Could you check a few things on this model? Use its own coordinates, in mm. A direction names the side the tool comes from. Give positions to 0.01 mm unless a question says otherwise; leave off trailing zeros. Order: outer loops, then holes, each group sorted by start corner. A loop starts at its lowest first (then second) coordinate and runs counter-clockwise, first axis right, second up. Notation, with made-up numbers: M -7.5,76 L 4.5,76 A17 cw 4.5,92 Z; hole C 21,-10.5 d6. An arc over 180 degrees is marked long. Use a Markdown table: item, result. Add a question column.
```python
from build123d import *

# Parameters (mm, degrees)
F2_W      = 19
F2_H      = 44
F3_DEPTH  = 23
F3_FACE_W = 19
F3_FACE_H = 44
F4_DEPTH  = 5
F5_R      = 17
F6_T      = -1
F7_R      = 9
F8_DEPTH  = 1
F9_R      = 9
F10_DEPTH = 0.5
F11_R     = 9
F12_DEPTH = 0.5
F14_DEPTH = 25


with BuildPart() as f3:
    # F2 (on offset) → F3 (new body)
    with BuildSketch(Plane.XZ.offset(-25)):
        Rectangle(F2_W, F2_H)
    extrude(amount=F3_DEPTH)

    # F3_face (on face) → F4 (join)
    with BuildSketch(Plane(origin=(0, 25, 0), x_dir=(1, 0, 0), z_dir=(0, 1, 0))):
        Rectangle(F3_FACE_W, F3_FACE_H)
    extrude(amount=F4_DEPTH)

    # F5
    f5_edges = [f3.edges().sort_by_distance(p)[0] for p in [
        (0, 2, 22),
        (0, 2, -22),
    ]]
    fillet(f5_edges, radius=F5_R)

    # F6
    f6_openings = [f3.faces().sort_by_distance(p)[0] for p in [
        (0, 30, 0),
    ]]
    offset(amount=F6_T, openings=f6_openings)

    # F7 (on face) → F8 (cut, symmetric)
    with BuildSketch(Plane(origin=(0, 3, 0), x_dir=(-1, 0, 0), z_dir=(0, 1, 0))):
        Circle(F7_R)
    extrude(amount=F8_DEPTH, both=True, mode=Mode.SUBTRACT)

    # F9 (on face) → F10 (cut)
    with BuildSketch(Plane.YZ.offset(9.5)):
        with Locations((30, 0)):
            Circle(F9_R)
    extrude(amount=-F10_DEPTH, mode=Mode.SUBTRACT)

    # F11 (on face) → F12 (cut)
    with BuildSketch(Plane(origin=(-9.5, 0, 0), x_dir=(0, -1, 0), z_dir=(-1, 0, 0))):
        with Locations((-30, 0)):
            Circle(F11_R)
    extrude(amount=-F12_DEPTH, mode=Mode.SUBTRACT)

    # F13 (on face) → F14 (cut)
    with BuildSketch(Plane(origin=(-9, 0, 0), x_dir=(0, -1, 0), z_dir=(-1, 0, 0))):
        with BuildLine():
            Line((-24, 2), (-24, -2))
            ThreePointArc((-24, -2), (-22, 0), (-24, 2))
        make_face()
    extrude(amount=-F14_DEPTH, mode=Mode.SUBTRACT)


solid = f3.part
```
1) Please list where these lines run through material, in increasing order: line 1 (X direction, y = 3.55, z = 0); line 2 (X direction, y = 9.5, z = 3); line 3 (Z direction, x = -4.5, y = 25.25). Write a range as from..to.
2) For pin 1 (0.5 mm diameter, centred on x = -8, z = 4, fed in from +Y); pin 2 (2 mm diameter, centred on x = -6, z = -11, fed in from -Y); pin 3 (2 mm diameter, centred on x = 7, y = 6.5, fed in from +Z); pin 4 (11 mm diameter, centred on x = 0, z = 0, fed in from -Y), each with a flat end and sliding along its axis, tell me the tip position at first contact or that it passes through.
3) For faces 1 (the face through (-8.2, 3, -4.4)), 2 (the face through (-9.254, 21.002, -0.198)), 3 (the face through (9.254, 21.002, 0.198)), which set-ups out of +Z, -Z, +X, -X, +Y, -Y let a thin tool reach every point of the face, with its end or its side?
4) Suppose I cut it at C-C on y = 25. Please give me the cut outline in (x, z), and give its area (3 significant figures).
5) Suppose I cut it at A-A on z = 0. Please give me the cut outline in (x, y).
6) Suppose I cut it at B-B on x = 0. Please give me the cut outline in (y, z).
7) Suppose I cut it at D-D on z = 7. Please give me the cut outline in (x, y).
8) We'd pull the mould along Z, two halves only. Please class faces 4 (the face through (0.13, 6.85, -16.89)), 5 (the face through (9.15, 2, 0.07)), 6 (the face through (9, 26, 0)): pulls with the +Z half, pulls with the -Z half, needs draft (parallel to the pull), parting line crosses it, or undercut.
Values found:
| question | item | result |
|---|---|---|
| 1 | line 1 | x = -9.5..-9, 9..9.5 |
| 1 | line 2 | x = -9.5..-8.5, 8.5..9.5 |
| 1 | line 3 | z = -22..-21, 21..22 |
| 2 | pin 1 | stops at y = 3 |
| 2 | pin 2 | stops at y = 2.75 |
| 2 | pin 3 | stops at z = 17.52 |
| 2 | pin 4 | passes through |
| 3 | face 1 | +Y |
| 3 | face 2 | -X, +Y |
| 3 | face 3 | +X, +Y |
| 4 | outline | M -9.5,-22 L 9.5,-22 L 9.5,-7.48 L 9,-7.48 L 9,7.48 L 9.5,7.48 L 9.5,22 L -9.5,22 L -9.5,7.48 L -9,7.48 L -9,-7.48 L -9.5,-7.48 Z; hole M -8.5,-21 L 8.5,-21 L 8.5,21 L -8.5,21 Z |
| 4 | area | 107 mm^2 |
| 5 | outline | M -9.5,2 L -9,2 L -9,4 L -8.5,4 L -8.5,22 L -9,22 L -9,21 L -9.5,21 Z; M -9,24 L -8.5,24 L -8.5,30 L -9,30 Z; M 8.5,4 L 9,4 L 9,2 L 9.5,2 L 9.5,21 L 9,21 L 9,22 L 8.5,22 Z; M 8.5,24 L 9,24 L 9,30 L 8.5,30 Z |
| 6 | outline | M 2.48,-9 A17 ccw 19,-22 L 30,-22 L 30,-21 L 19,-21 A16 cw 3.51,-9 Z; M 2.48,9 L 3.51,9 A16 cw 19,21 L 30,21 L 30,22 L 19,22 A17 ccw Z |
| 7 | outline | M -9.5,2.12 L -5.66,2.12 L -5.66,3.13 L -8.5,3.13 L -8.5,30 L -9,30 L -9,24.34 L -9.5,24.34 Z; M 5.66,2.12 L 9.5,2.12 L 9.5,24.34 L 9,24.34 L 9,30 L 8.5,30 L 8.5,3.13 L 5.66,3.13 Z |
| 8 | face 4 | pulls with the -Z half |
| 8 | face 5 | needs draft |
| 8 | face 6 | undercut |
